Autodesk Inventor part; units mm, degrees
ref_plane "Work Plane1" through (0, 0, 0) normal (0, 0, 1) x (1, 0, 0)
ref_plane "Work Plane2" through (0, 0, 4) normal (0, 0, -1) x (-1, 0, 0)
ref_plane "Work Plane3" through (-20.3, -49, 28.5) normal (0, -1, 0) x (1, 0, 0)
ref_plane "Work Plane1" through (0, 0, 0) normal (0, 0, 1) x (1, 0, 0)
sketch "Sketch1" plane through (0, 0, 0) normal (0, 0, 1) x (1, 0, 0)
  circle A0 centre (-17.3, 4) radius 1.35
  circle A1 centre (-17.3, -18) radius 1.35
  circle A2 centre (-17.3, -40) radius 1.35
  line L0 (-17.3, 4) -> (-14.8, 4)
  line L1 (-14.8, 4) -> (-14.8, 9)
  line L2 (-14.8, 9) -> (-20.3, 9)
  line L3 (-17.3, -40) -> (-17.3, -54)
  line L4 (-14.8, 4) -> (-14.8, -54)
  line L5 (-14.8, -54) -> (-17.3, -54)
  line L6 (-17.3, -54) -> (-20.3, -54)
  line L7 (-20.3, -54) -> (-20.3, 9)
  point P0 (0, 0)
  dimension "d0" = 2.5
  dimension "d1" = 5
  dimension "d2" = 5.5
  dimension "d3" = 14
extrude "Extrusion1" add sketch "Sketch1" along normal blind 36.5
sketch "Sketch2" plane through (-20.3, -54, 0) normal (0, -1, 0) x (1, 0, 0)
  line L0 (0, 0) -> (5.5, 0)
  line L1 (5.5, 0) -> (5.5, 36.5)
  line L2 (0, 36.5) -> (5.5, 36.5)
  line L3 (0, 0) -> (0, 36.5)
  line L4 (2.75, 36.5) -> (2.75, 25.5)
  circle A0 centre (2.75, 25.5) radius 1.5
  point P0 (20.3, 0)
  dimension "d6" = 11
  dimension "d7" = 3
extrude "Extrusion2" cut sketch "Sketch2" against normal blind 10 contours A0
sketch "Sketch3" plane through (-20.3, -54, 0) normal (-1, 0, 0) x (0, 0, 1)
  line L0 (0, 63) -> (0, 0)
  line L1 (0, 0) -> (36.5, 0)
  line L2 (36.5, 63) -> (36.5, 0)
  line L3 (0, 63) -> (36.5, 63)
  line L4 (0, 0) -> (36.5, 0)
  line L5 (36.5, 0) -> (28.5, 0)
  line L6 (28.5, 0) -> (28.5, 8)
  line L7 (28.5, 8) -> (36.5, 8)
  line L8 (36.5, 8) -> (36.5, 0)
  point P0 (0, 54)
  dimension "d10" = 8
  dimension "d11" = 8
extrude "Extrusion3" cut sketch "Sketch3" against normal blind 10 contours L6 L7 L2 L1
sketch "Sketch4" plane through (-20.3, 9, 0) normal (0, 1, 0) x (1, 0, 0)
  line L0 (5.5, 0) -> (0, 0)
  line L1 (0, 0) -> (0, -36.5)
  line L2 (5.5, -36.5) -> (0, -36.5)
  line L3 (5.5, 0) -> (5.5, -36.5)
  line L4 (6.8, -6) -> (8.8, -6)
  line L5 (6.8, -6) -> (5.5, -6)
  line L6 (5.5, -6) -> (5.5, -6.5)
  line L7 (5.5, 0) -> (5.5, -28.5)
  line L8 (5.5, -6.5) -> (15.5, -6.5)
  line L9 (15.5, -6.5) -> (15.5, -11.5)
  line L10 (15.5, -11.5) -> (5.5, -11.5)
  line L11 (5.5, -11.5) -> (5.5, -6.5)
  point P0 (20.3, 0)
  dimension "d14" = 0.5
  dimension "d15" = 10
  dimension "d16" = 5
extrude "Extrusion4" add sketch "Sketch4" against normal up to surface (63 mm away) contours L8 L9 L10 L3
sketch "Sketch5" plane through (-4.8, 9, 6.5) normal (0, 0, -1) x (-1, 0, 0)
  circle A0 centre (12.5, -49) radius 1.35
  circle A1 centre (12.5, -27) radius 1.35
  circle A2 centre (12.5, -5) radius 1.35
  line L0 (10, -63) -> (10, 0)
  line L1 (15.5, -63) -> (10, -63)
  line L2 (15.5, 0) -> (15.5, -63)
  line L3 (10, 0) -> (15.5, 0)
  line L4 (0, -63) -> (10, -63)
  line L5 (10, 0) -> (10, -63)
  line L6 (0, 0) -> (10, 0)
  line L7 (0, 0) -> (0, -63)
  line L8 (-19.8, 5.5) -> (-16.3, 5.5)
  line L9 (-19.8, 5.5) -> (-24.9, -0.5)
  line L10 (-24.9, -0.5) -> (-24.9, -53.6)
  line L11 (-24.9, -53.6) -> (-19.8, -59.6)
  line L12 (-19.8, -59.6) -> (10.2, -59.6)
  line L13 (10.2, -59.6) -> (15.3, -53.6)
  line L14 (15.3, -53.6) -> (15.3, -0.5)
  line L15 (15.3, -0.5) -> (10.2, 5.5)
  line L16 (6.7, 5.5) -> (10.2, 5.5)
  arc A3 (9.7, 2.5) -> (6.7, 5.5) centre (6.7, 2.5) ccw
  line L17 (9.7, -51) -> (9.7, 2.5)
  arc A4 (6.7, -54) -> (9.7, -51) centre (6.7, -51) ccw
  line L18 (-16.3, -54) -> (6.7, -54)
  arc A5 (-19.3, -51) -> (-16.3, -54) centre (-16.3, -51) ccw
  line L19 (-19.3, 2.5) -> (-19.3, -51)
  arc A6 (-16.3, 5.5) -> (-19.3, 2.5) centre (-16.3, 2.5) ccw
  circle A7 centre (12.5, -5) radius 1.35
  circle A8 centre (12.5, -27) radius 1.35
  circle A9 centre (12.5, -49) radius 1.35
  circle A10 centre (6.2, -56.8) radius 1.35
  circle A11 centre (-22.1, -5) radius 1.35
  circle A12 centre (-22.1, -27) radius 1.35
  circle A13 centre (-22.1, -49) radius 1.35
  circle A14 centre (-15.8, -56.8) radius 1.35
  line L20 (10, 0) -> (10, -63)
  line L21 (10, -63) -> (0, -63)
  line L22 (0, -63) -> (0, -54.5)
  line L23 (0, -54.5) -> (10, -54.5)
  line L24 (10, -54.5) -> (10, -63)
  point P0 (-4.8, -9)
  dimension "d19" = 10
  dimension "d20" = 8.5
extrude "Extrusion5" add sketch "Sketch5" along normal up to surface (6.5 mm away) contours L0 L12 L7 L23 | L0 L4 L7 L12
ref_plane "Work Plane2" through (0, 0, 4) normal (0, 0, -1) x (-1, 0, 0)
sketch "Sketch6" plane through (0, 0, 4) normal (0, 0, -1) x (-1, 0, 0)
  circle A0 centre (17.3, 4) radius 1.35
  circle A1 centre (17.3, -18) radius 1.35
  circle A2 centre (11, -47.8) radius 1.35
  circle A3 centre (17.3, -40) radius 1.35
  circle A4 centre (17.3, -18) radius 1.35
  circle A5 centre (17.3, 4) radius 1.35
  line L0 (20.3, -54) -> (4.8, -54)
  line L1 (20.3, 9) -> (20.3, -54)
  line L2 (14.8, 9) -> (20.3, 9)
  line L3 (14.8, -45.5) -> (14.8, 9)
  line L4 (14.8, -45.5) -> (4.8, -45.5)
  line L5 (4.8, -45.5) -> (4.8, -54)
  circle A6 centre (11, -47.8) radius 1.35
  circle A7 centre (11, -47.8) radius 1.35
  line L6 (17.3, 4) -> (17.3, 6.6)
  line L7 (18.8011, 6.6) -> (20.3022, 4)
  line L8 (20.3022, 4) -> (18.8011, 1.4)
  line L9 (18.8011, 1.4) -> (15.7989, 1.4)
  line L10 (15.7989, 1.4) -> (14.2978, 4)
  line L11 (14.2978, 4) -> (15.7989, 6.6)
  line L12 (15.7989, 6.6) -> (18.8011, 6.6)
  line L13 (18.8011, 1.4) -> (28.5961, 1.4)
  line L14 (28.5961, 1.4) -> (28.5961, 6.6)
  line L15 (28.5961, 6.6) -> (18.8011, 6.6)
  line L16 (18.8011, 6.6) -> (18.8011, 1.4)
  line L17 (11, -47.8) -> (13.6, -47.8)
  line L18 (13.6, -49.3011) -> (11, -50.8022)
  line L19 (11, -50.8022) -> (8.4, -49.3011)
  line L20 (8.4, -49.3011) -> (8.4, -46.2989)
  line L21 (8.4, -46.2989) -> (11, -44.7978)
  line L22 (11, -44.7978) -> (13.6, -46.2989)
  line L23 (13.6, -46.2989) -> (13.6, -49.3011)
  line L24 (13.6, -49.3011) -> (8.4, -49.3011)
  line L25 (8.4, -49.3011) -> (8.4, -56.2377)
  line L26 (8.4, -56.2377) -> (13.6, -56.2377)
  line L27 (13.6, -56.2377) -> (13.6, -49.3011)
  line L28 (18.8011, -15.4) -> (20.3022, -18)
  line L29 (20.3022, -18) -> (18.8011, -20.6)
  line L30 (18.8011, -20.6) -> (28.5961, -20.6)
  line L31 (28.5961, -20.6) -> (28.5961, -15.4)
  line L32 (28.5961, -15.4) -> (18.8011, -15.4)
  line L33 (18.8011, -15.4) -> (18.8011, -20.6)
  line L34 (17.3, -18) -> (17.3, -15.4)
  line L35 (18.8011, -20.6) -> (15.7989, -20.6)
  line L36 (15.7989, -15.4) -> (18.8011, -15.4)
  line L37 (15.7989, -20.6) -> (14.2978, -18)
  line L38 (14.2978, -18) -> (15.7989, -15.4)
  line L39 (18.8011, -37.4) -> (20.3022, -40)
  line L40 (20.3022, -40) -> (18.8011, -42.6)
  line L41 (18.8011, -42.6) -> (28.5961, -42.6)
  line L42 (28.5961, -42.6) -> (28.5961, -37.4)
  line L43 (28.5961, -37.4) -> (18.8011, -37.4)
  line L44 (18.8011, -37.4) -> (18.8011, -42.6)
  line L45 (17.3, -40) -> (17.3, -37.4)
  line L46 (18.8011, -42.6) -> (15.7989, -42.6)
  line L47 (15.7989, -37.4) -> (18.8011, -37.4)
  line L48 (15.7989, -42.6) -> (14.2978, -40)
  line L49 (14.2978, -40) -> (15.7989, -37.4)
  point P0 (0, 0)
  dimension "d24" = 2.6
  dimension "d25" = 2.6
  dimension "d28" = 22
extrude "Extrusion6" cut sketch "Sketch6" against normal blind 3 contours L12 L16 L9 L10 L3 L11 | L15 L1 L7 | L7 L8 L16 | L3 L10 L11 | L1 L15 L14 L13 | L1 L13 L8 | L38 L36 L33 L35 L37 L3 | L3 L37 L38 | L32 L31 L30 L1 | L1 L28 L32 | L29 L33 L28 | L1 L30 L29 | L49 L47 L44 L46 L48 L3 | L3 L48 L49 | L43 L42 L41 L1 | L1 L39 L43 | L40 L44 L39 | L1 L41 L40 | A2 | L22 L23 L24 L20 L21 L4 | L4 L21 L22 | L27 L26 L25 L0 | L0 L25 L19 L18 L27 | L24 L18 L19
sketch "Sketch7" plane through (0, 0, 36.5) normal (0, 0, 1) x (1, 0, 0)
  line L0 (-20.3, -46) -> (-14.8, -46)
  line L1 (-14.8, -46) -> (-14.8, 9)
  line L2 (-14.8, 9) -> (-20.3, 9)
  line L3 (-20.3, 9) -> (-20.3, -46)
  circle A0 centre (-17.3, 4) radius 1.35
  circle A1 centre (-17.3, -18) radius 1.35
  circle A2 centre (-17.3, -40) radius 1.35
  point P0 (0, 0)
extrude "Extrusion7" add sketch "Sketch7" against normal blind 25 contours A0 | A1 | A2
ref_plane "Work Plane3" through (-20.3, -49, 28.5) normal (0, -1, 0) x (1, 0, 0)
sketch "Sketch8" plane through (-20.3, -49, 28.5) normal (0, -1, 0) x (1, 0, 0)
  circle A0 centre (2.75, -3) radius 1.5
  line L0 (2.75, -3) -> (2.75, -0.4)
  line L1 (4.2511, -0.4) -> (5.7522, -3)
  line L2 (5.7522, -3) -> (4.2511, -5.6)
  line L3 (4.2511, -5.6) -> (1.2489, -5.6)
  line L4 (1.2489, -5.6) -> (-0.2522, -3)
  line L5 (-0.2522, -3) -> (1.2489, -0.4)
  line L6 (1.2489, -0.4) -> (4.2511, -0.4)
  line L7 (1.2489, -0.4) -> (-2.7612, -0.4)
  line L8 (-2.7612, -0.4) -> (-2.7612, -5.6)
  line L9 (-2.7612, -5.6) -> (1.2489, -5.6)
  line L10 (1.2489, -5.6) -> (1.2489, -0.4)
  point P0 (20.3, -28.5)
  dimension "d38" = 2.6
extrude "Extrusion8" cut sketch "Sketch8" against normal blind 3 contours A0 L0 L6 L1 L2 L3 L10 | A0 L10 L6 L0 | L10 L4 L5 | L9 L8 L7 L5 L4
sketch "Sketch9" plane through (-20.3, 9, 0) normal (0, 1, 0) x (1, 0, 0)
  line L0 (5.5, 0) -> (0, 0)
  line L1 (0, 0) -> (0, -36.5)
  line L2 (5.5, -36.5) -> (0, -36.5)
  line L3 (5.5, -11.5) -> (5.5, -36.5)
  line L4 (5.5, -11.5) -> (15.5, -11.5)
  line L5 (15.5, -11.5) -> (15.5, -6.5)
  line L6 (15.5, -6.5) -> (5.5, -6.5)
  line L7 (5.5, 0) -> (5.5, -6.5)
  line L8 (5.5, -11.5) -> (15.5, -11.5)
  line L9 (5.5, -11.5) -> (5.5, -28.5)
  line L10 (15.5, -11.5) -> (5.5, -11.5)
  line L11 (5.5, -20) -> (15.5, -20)
  line L12 (5.5, -20) -> (11.5, -20)
  line L13 (5.5, -24) -> (5.5, -20)
  line L14 (15.5, -24) -> (15.5, -27)
  line L15 (15.5, -27) -> (5.5, -27)
  line L16 (5.5, -27) -> (5.5, -24)
  line L17 (5.5, -11.5) -> (15.5, -11.5)
  line L18 (15.5, -11.5) -> (15.5, -16)
  line L19 (15.5, -16) -> (5.5, -16)
  line L20 (5.5, -16) -> (5.5, -11.5)
  line L21 (5.5, -16) -> (11.5, -16)
  line L22 (11.5, -16) -> (11.5, -20)
  line L23 (11.5, -20) -> (5.5, -20)
  line L24 (5.5, -20) -> (5.5, -16)
  line L25 (5.5, -20) -> (15.5, -20)
  line L26 (15.5, -20) -> (15.5, -27)
  line L27 (15.5, -27) -> (5.5, -27)
  line L28 (5.5, -27) -> (5.5, -20)
  point P0 (20.3, 0)
  dimension "d41" = 8.5
  dimension "d44" = 10
  dimension "d45" = 3
  dimension "d48" = 4.5
extrude "Extrusion9" add sketch "Sketch9" against normal up to surface (63 mm away) contours L18 L19 L3 L4 | L3 L11 L26 L14 L15 | L19 L22 L11 L3
sketch "Sketch11" plane through (-20.3, -54, 28.5) normal (0, 0, 1) x (1, 0, 0)
  line L0 (5.5, 8) -> (5.5, 0)
  line L1 (0, 8) -> (5.5, 8)
  line L2 (0, 0) -> (0, 8)
  line L3 (5.5, 0) -> (0, 0)
  point P0 (20.3, 54)
extrude "Extrusion10" add sketch "Sketch11" along normal blind 2
sketch "Sketch12" plane through (-20.3, -54, 0) normal (0, -1, 0) x (1, 0, 0)
  line L0 (0, 0) -> (0, 30.5)
  line L1 (0, 21.5909) -> (7, 21.5909)
  line L2 (7, 21.5909) -> (7, 7.5909)
  line L3 (7, 7.5909) -> (0, 7.5909)
  line L4 (0, 7.5909) -> (0, 21.5909)
  point P0 (20.3, 0)
  dimension "d51" = 7
  dimension "d52" = 14
extrude "Extrusion11" cut sketch "Sketch12" against normal through all
properties part number "side"
Build history of the part. All positions in model axes, mm. A direction names the side the tool comes from. Coordinates: 2 decimals unless noted, no trailing zeros. Write each loop counter-clockwise with the first axis right and the second up, starting at its lowest first coordinate (ties: lowest second). Pieces come first, ordered by that corner, then holes.
(1) Cut at C-C on z = 29.5. List the corners of the cut face in (x, y), and give its area (4 significant figures).
(2) 3-axis set-ups, long thin cutter, end or side, ignore diameter. For faces 1 (the flat face through (-7, -22, 20)), 2 (the flat face through (-8.4, -50, 5)), 3 (the flat face through (-15.43, -47.52, 27.03)): which of +Z, -Z, +X, -X, +Y, -Y reach the whole face in a straight line?
(3) Cut at B-B on y = -23.5. List the corners of the cut face in (x, z), and give its area (3 significant figures).
(4) Pin check, flat tips, straight feed: pin 1 Ø2 at (x, y) = (-11, -47.8) entering from +Z; pin 2 Ø2.5 at (x, y) = (-17.3, 4) entering from -Z; pin 3 Ø3 at (y, z) = (-35.5, 11.5) entering from -X. Stop position of each tip, or through.
(5) Cut at A-A on z = 3. List the corners of the cut face in (x, y).
(6) Drill centre lines: line 1 (Y direction, x = -17.3, z = 1.35); line 2 (Z direction, x = -19.5, y = -18); line 3 (X direction, y = -44.6, z = 25.5). Where is each one in solid material? Low to high.
(7) Mould opens along Z. For faces 4 (the flat face through (-4.8, -22, 23)), 5 (the flat face through (-18, -50, 30.5)), 6 (the flat face through (-15.226, 2.393, 5.479)) say: pulls with the +Z half, pulls with the -Z half, needs draft (parallel to the pull), parting line crosses it, or undercut.
Working result:
1. outline: (-20.3, -54) - (-14.8, -54) - (-14.8, 9) - (-20.3, 9) - close
1. area: 346.5 mm2
2. face 1: +X, +Y, -Y
2. face 2: -Y
2. face 3: -X
3. outline: (-20.3, 0) - (-14.8, 0) - (-14.8, 6.5) - (-4.8, 6.5) - (-4.8, 16) - (-8.8, 16) - (-8.8, 20) - (-4.8, 20) - (-4.8, 27) - (-14.8, 27) - (-14.8, 36.5) - (-20.3, 36.5) - (-20.3, 21.59) - (-13.3, 21.59) - (-13.3, 7.59) - (-20.3, 7.59) - close
3. area: 292 mm2
4. pin 1: stops at z = 27
4. pin 2: stops at z = 21.59
4. pin 3: stops at x = -13.3
5. outline: (-20.3, -54) - (-4.8, -54) - (-4.8, -45.5) - (-14.8, -45.5) - (-14.8, 9) - (-20.3, 9) - close; hole circle Ø2.7 at (-17.3, -40); hole circle Ø2.7 at (-17.3, -18); hole circle Ø2.7 at (-17.3, 4); hole circle Ø2.7 at (-11, -47.8)
6. line 1: y = -54 to -41.35, -38.65 to -19.35, -16.65 to 2.65, 5.35 to 9
6. line 2: z = 0 to 4, 7 to 7.59, 21.59 to 36.5
6. line 3: x = -20.3 to -19.05, -16.05 to -4.8
7. face 4: needs draft
7. face 5: pulls with the +Z half
7. face 6: undercut
